Verification items for the finished model (mm, model axes). Give positions to 0.01 mm unless a question says otherwise; leave off trailing zeros. Loops run counter-clockwise (first coordinate to the right, second up) from the corner with the lowest first, then second, coordinate; pieces in that order, holes last. Notation, with made-up numbers: (67.5, 26) - (83.5, 26) arc R17 cw to (83.5, 38) - close; hole circle Ø8 at (53.5, 35). An arc over 180 degrees is marked (long way). One line per item, written item: value. Start each with the question number.
1. Mould release check, pull along Y, two halves, no side actions. Record for faces 1 (the cylindrical face through (-94.613, 13.574, 1.565)), 2 (the flat face through (-36, 1, 3.175)), 3 (the cylindrical face through (-109.22, 39.46, 1.57)): pulls with the +Y half, pulls with the -Y half, needs draft (parallel to the pull), parting line crosses it, or undercut.
2. Sectioned sample at B-B (x = 9). Record the cut outline in (y, z) (3 decimals).
3. Scan lines: L1, parallel to X at y = -15.5, z = 1.4 (3 decimals); L2, parallel to Y at x = 19, z = 0.35; L3, parallel to X at y = 18, z = 0.65 (3 decimals). Record each from-to range of solid material in increasing order. Write a range as [from, to].
4. Sectioned sample at A-A (z = 1.2). Record the cut outline in (x, y) (3 decimals), plus the area to 3 significant figures.
5. Sectioned sample at C-C (y = 28.5). Record the cut outline in (x, z) (3 decimals), plus the area to 3 significant figures.
from build123d import *

# Parameters (mm, degrees)
F0_R     = 2.54
F1_DEPTH = 3.175


# Not quite as in the source:
# - a feature names something its author has since deleted; it is built from what else it names


with BuildPart() as f1:
    # F0 (on Top) → F1 (new body)
    with BuildSketch(Plane.XY):
        with BuildLine():
            ThreePointArc((-41.275, 0), (-29.1858323935, 29.1858323935), (0, 41.275))
            Line((0, 41.275), (-104.775, 41.275))
            ThreePointArc((-104.775, 41.275), (-109.2651280605, 39.4151280605), (-111.125, 34.925))
            Line((-111.125, 34.925), (-111.125, 0))
            Line((-111.125, 0), (-41.275, 0))
        make_face()
        with Locations((-92.075, 13.462)):
            Circle(F0_R, mode=Mode.SUBTRACT)
        with BuildLine():
            Line((-104.775, -41.275), (0, -41.275))
            ThreePointArc((0, -41.275), (-29.1858323935, -29.1858323935), (-41.275, 0))
            Line((-41.275, 0), (-111.125, 0))
            Line((-111.125, 0), (-111.125, -34.925))
            ThreePointArc((-111.125, -34.925), (-109.2651280605, -39.4151280605), (-104.775, -41.275))
        make_face()
        with Locations((-92.075, -13.462)):
            Circle(F0_R, mode=Mode.SUBTRACT)
        with BuildLine():
            Line((0, 2.8299858928), (0, 41.275))
            ThreePointArc((0, 41.275), (-29.1858323935, 29.1858323935), (-41.275, 0))
            Line((-41.275, 0), (0, 0))
            Line((0, 0), (0, 2.8299858928))
        make_face()
        with BuildLine():
            ThreePointArc((-13.3722019973, 17.6013019973), (-13.6941230664, 15.9828954935), (-14.610876709, 14.610876709))
            ThreePointArc((-14.610876709, 14.610876709), (-21.5084809282, 19.2197085011), (-13.3722019973, 17.6013019973))
        make_face(mode=Mode.SUBTRACT)
        with BuildLine():
            ThreePointArc((-41.275, 0), (-29.1858323935, -29.1858323935), (0, -41.275))
            Line((0, -41.275), (0, 0))
            Line((0, 0), (-41.275, 0))
        make_face()
        with BuildLine():
            ThreePointArc((-13.3722019973, -17.6013019973), (-21.5084809282, -19.2197085011), (-14.610876709, -14.610876709))
            ThreePointArc((-14.610876709, -14.610876709), (-13.6941230664, -15.9828954935), (-13.3722019973, -17.6013019973))
        make_face(mode=Mode.SUBTRACT)
        with BuildLine():
            ThreePointArc((0, -41.275), (29.1858323935, -29.1858323935), (41.275, 0))
            ThreePointArc((41.275, 0), (29.1858323935, 29.1858323935), (0, 41.275))
            Line((0, 41.275), (0, 2.8299858928))
            Line((0, 2.8299858928), (0, 0))
            Line((0, 0), (0, -41.275))
        make_face()
        with BuildLine():
            ThreePointArc((21.8304019973, -17.6013019973), (15.9828954935, -21.5084809282), (14.610876709, -14.610876709))
            ThreePointArc((14.610876709, -14.610876709), (19.2197085011, -13.6941230664), (21.8304019973, -17.6013019973))
        make_face(mode=Mode.SUBTRACT)
        with BuildLine():
            ThreePointArc((21.8304019973, 17.6013019973), (19.2197085011, 13.6941230664), (14.610876709, 14.610876709))
            ThreePointArc((14.610876709, 14.610876709), (15.9828954935, 21.5084809282), (21.8304019973, 17.6013019973))
        make_face(mode=Mode.SUBTRACT)
    extrude(amount=F1_DEPTH)


solid = f1.part
Results are:
1. face 1: undercut
1. face 2: needs draft
1. face 3: pulls with the +Y half
2. outline: (-40.282, 0) - (40.282, 0) - (40.282, 3.175) - (-40.282, 3.175) - close
3. L1: x = [-111.125, -93.591], [-90.559, -21.271], [-13.931, 13.931], [21.271, 38.254]
3. L2: y = [-36.64, -21.59], [-13.61, 13.61], [21.59, 36.64]
3. L3: x = [-111.125, -21.812], [-13.391, 13.391], [21.812, 37.143]
4. outline: (-111.125, -34.925) arc R6.35 ccw to (-104.775, -41.275) - (0, -41.275) arc R41.275 ccw to (0, 41.275) - (-104.775, 41.275) arc R6.35 ccw to (-111.125, 34.925) - close; hole circle Ø5.08 at (-92.075, -13.462); hole circle Ø5.08 at (-92.075, 13.462); hole circle Ø8.458 at (-17.601, -17.601); hole circle Ø8.458 at (-17.601, 17.601); hole circle Ø8.458 at (17.601, -17.601); hole circle Ø8.458 at (17.601, 17.601)
4. area: 11,600 mm^2
5. outline: (-111.125, 0) - (29.856, 0) - (29.856, 3.175) - (-111.125, 3.175) - close
5. area: 448 mm^2
